Job drawing, mm, ordinate dimensions from the low corner. One solid piece. Round coordinates to 2 decimals unless told otherwise and drop trailing zeros. Loops run counter-clockwise (first coordinate to the right, second up) from the corner with the lowest first, then second, coordinate; pieces in that order, holes last. Notation, with made-up numbers: M 67,22.25 L 106,22.25 A33 ccw 106,55.25 Z; hole C 43,-18.75 d1. An arc over 180 degrees is marked long. Use a Markdown table: item, result. Add a question column.
(1) Wall check: L1, parallel to Z at x = 4.75, y = 200; L2, parallel to Y at x = 4.5, z = 173. Give the ranges that are in metal, low to high.
(2) Flat gauge pin, fed straight in: P1, Ø4, axis at y = 499, z = 254.5, coming from the -X side. Where does the tip first touch, or does it go through?
(3) Band-saw the part on B-B, the plane z = 40. Write the cut outline in (x, y).
(4) Band-saw the part on A-A, the plane y = 400. Write the cut outline in (x, z).
(5) Band-saw the part on C-C, the plane y = 332.5. Write the cut outline in (x, z).
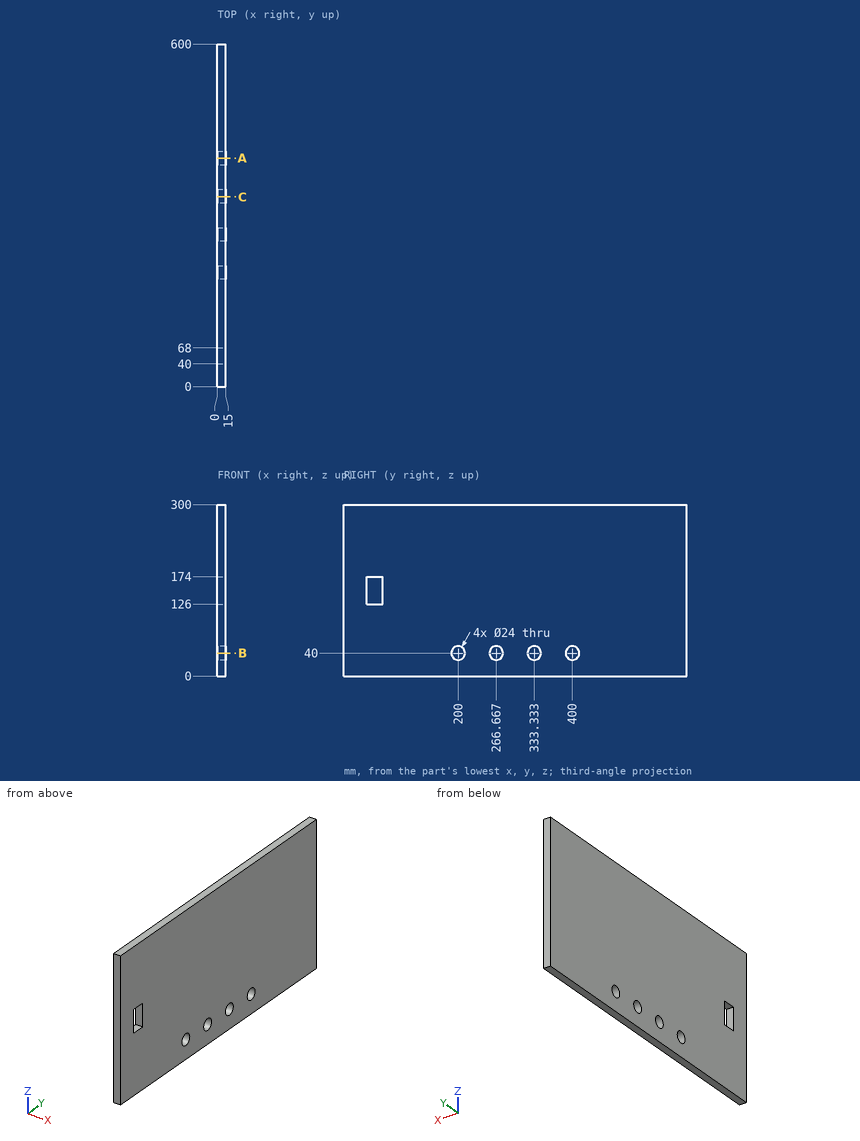
Return value:
| question | item | result |
|---|---|---|
| 1 | L1 | 0 to 28, 52 to 300 |
| 1 | L2 | 0 to 40, 68 to 600 |
| 2 | P1 | x = 0 |
| 3 | outline | M 0,0 L 15,0 L 15,188 L 0,188 Z; M 0,212 L 15,212 L 15,254.67 L 0,254.67 Z; M 0,278.67 L 15,278.67 L 15,321.33 L 0,321.33 Z; M 0,345.33 L 15,345.33 L 15,388 L 0,388 Z; M 0,412 L 15,412 L 15,600 L 0,600 Z |
| 4 | outline | M 0,0 L 15,0 L 15,28 L 0,28 Z; M 0,52 L 15,52 L 15,300 L 0,300 Z |
| 5 | outline | M 0,0 L 15,0 L 15,28.03 L 0,28.03 Z; M 0,51.97 L 15,51.97 L 15,300 L 0,300 Z |
